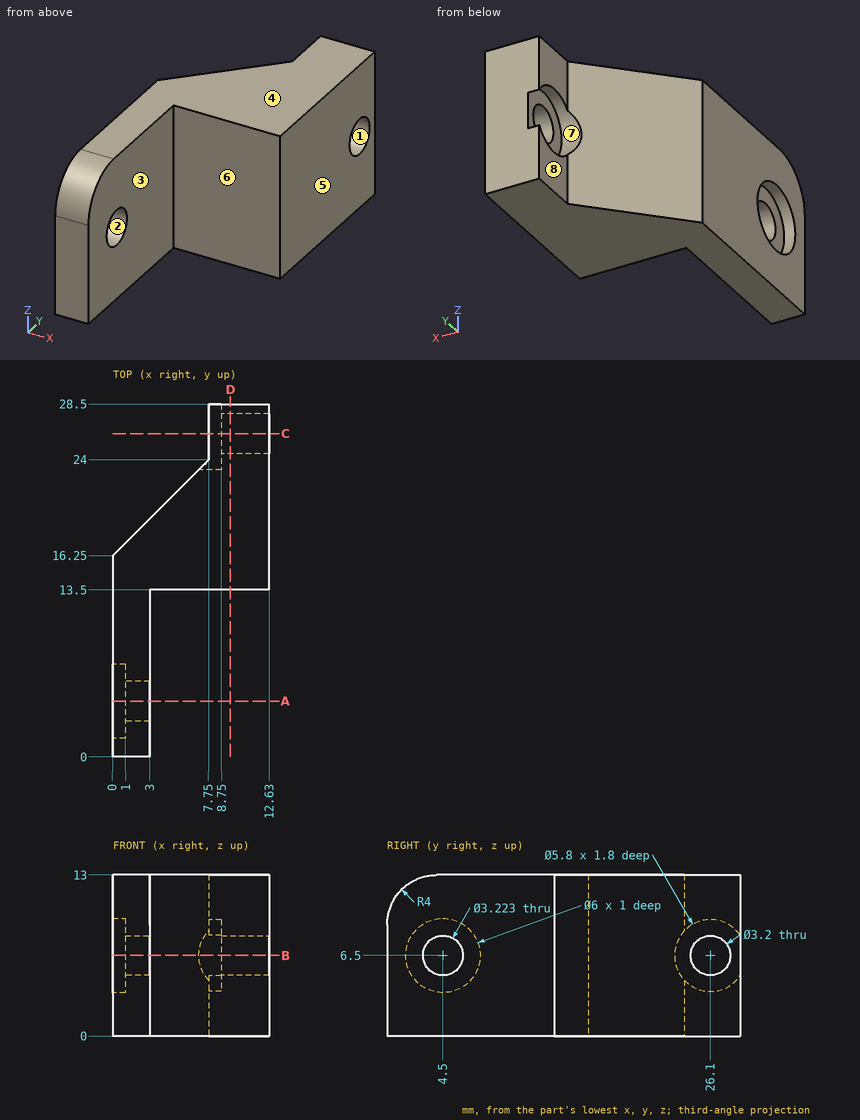
The figure shows three views and two pictorial views of one solid part (mm, origin at its lowest corner). Answer the questions. A direction names the side the tool comes from. Coordinates: 2 decimals unless noted, no trailing zeros. Write each loop counter-clockwise with the first axis right and the second up, starting at its lowest first coordinate (ties: lowest second). Pieces come first, ordered by that corner, then holes. Notation, with made-up numbers: (64, 9) -> (122, 9) arc R17 ccw to (122, 23) -> close; hole circle Ø9 at (34.25, 54). An arc over 180 degrees is marked (long way). Answer as a JSON object with one key per item and string values.
Q1. The part is cut by section C-C on y = 26.1. Give the vertices of the cut face in (x, z), then the cut area to 3 significant figures.
The answers:
{"outline": "(7.75, 0) -> (12.63, 0) -> (12.63, 4.9) -> (8.75, 4.9) -> (8.75, 3.6) -> (7.75, 3.6) -> close; (7.75, 9.4) -> (8.75, 9.4) -> (8.75, 8.1) -> (12.63, 8.1) -> (12.63, 13) -> (7.75, 13) -> close", "area": "45.2 mm2"}
Q2. Consider line 1 (Z direction, x = 8.15, y = 26.1); line 2 (Y direction, x = 10, z = 6.5); line 3 (X direction, y = 10.25, z = 1). Determine where each line is inside the solid, lowest interval first. Write a range as [from, to].
The answers:
{"line 1": "z = [0, 3.6], [9.4, 13]", "line 2": "y = [13.5, 24.5], [27.7, 28.5]", "line 3": "x = [0, 3]"}
Q3. Determine the mould class of the marked faces 1, 2, 3 and 4 for opening direction Z: pulls with the +Z half, pulls with the -Z half, needs draft (parallel to the pull), parting line crosses it, or undercut.
The answers:
{"face 1": "undercut", "face 2": "undercut", "face 3": "needs draft", "face 4": "pulls with the +Z half"}
Q4. Flat-ended cylindrical pins translate along their axes: pin 1 Ø4 at (y, z) = (26.1, 6.5) entering from +X; pin 2 Ø7.5 at (x, z) = (8, 3.5) entering from -Y; pin 3 Ø2.5 at (y, z) = (27, 6) entering from -X; pin 4 Ø1.9 at (y, z) = (4.5, 6.5) entering from +X. Find the tip coordinate at first contact, or state that the pin passes through.
The answers:
{"pin 1": "stops at x = 12.63", "pin 2": "stops at y = 13.5", "pin 3": "stops at x = 8.75", "pin 4": "passes through"}
Q5. A tool of negligible diameter and unlimited length cuts with its end or side. For the marked faces 5, 6, 7 and 8, from which of +Z, -Z, +X, -X, +Y, -Y can it reach the whole face along a straight path? Write none if from no direction.
The answers:
{"face 5": "+Z, -Z, +X, +Y, -Y", "face 6": "+Z, -Z, +X, -Y", "face 7": "-X", "face 8": "+Z, -Z, -X, +Y"}
Q6. The part is cut by section B-B on z = 6.5. Give the vertices of the cut face in (x, y).
The answers:
{"outline": "(0, 0) -> (3, 0) -> (3, 2.89) -> (1, 2.89) -> (1, 1.5) -> (0, 1.5) -> close; (0, 7.5) -> (1, 7.5) -> (1, 6.11) -> (3, 6.11) -> (3, 13.5) -> (12.63, 13.5) -> (12.63, 24.5) -> (8.75, 24.5) -> (8.75, 23.2) -> (6.95, 23.2) -> (0, 16.25) -> close; (8.75, 27.7) -> (12.63, 27.7) -> (12.63, 28.5) -> (8.75, 28.5) -> close"}
Q7. The part is cut by section A-A on y = 4.5. Give the vertices of the cut face in (x, z).
The answers:
{"outline": "(0, 0) -> (3, 0) -> (3, 4.89) -> (1, 4.89) -> (1, 3.5) -> (0, 3.5) -> close; (0, 9.5) -> (1, 9.5) -> (1, 8.11) -> (3, 8.11) -> (3, 13) -> (0, 13) -> close"}
Q8. The part is cut by section D-D on x = 9.5. Give the vertices of the cut face in (y, z), then the cut area to 3 significant figures.
The answers:
{"outline": "(13.5, 0) -> (28.5, 0) -> (28.5, 13) -> (13.5, 13) -> close; hole circle Ø3.2 at (26.1, 6.5)", "area": "187 mm2"}
